```python
from build123d import *

# Parameters (mm, degrees)
BOSS_EXTRUDE1_DEPTH             = 10
SKETCH2_W                       = 1.5
SKETCH2_H                       = 4.15
TAP_DRILL_FOR_M3X0_5_TAP1_D     = 2.5
TAP_DRILL_FOR_M3X0_5_TAP1_DEPTH = 8.248924226
TAP_DRILL_FOR_M3X0_5_TAP1_TIP   = 0.751075774
CHAMFER1_SIZE                   = 2


with BuildPart() as part:
    # Sketch1 → Boss-Extrude1 (new, symmetric)
    with BuildSketch(Plane(origin=(0, 0, 0), x_dir=(1, 0, 0), z_dir=(0, 1, 0))):
        with BuildLine():
            Line((-11.8, 0), (-16.8, 0))
            Line((-16.8, 0), (-16.8, 21.8))
            Line((-16.8, 21.8), (16.8, 21.8))
            Line((16.8, 21.8), (16.8, 0))
            Line((16.8, 0), (11.8, 0))
            ThreePointArc((11.8, 0), (0, 11.8), (-11.8, 0))
        make_face()
    extrude(amount=BOSS_EXTRUDE1_DEPTH, both=True)

    # Sketch2 → Cut-Revolve1 (revolve, cut)
    with BuildSketch(Plane.XY):
        with Locations((14.3, 5)):
            Rectangle(SKETCH2_W, SKETCH2_H)
        with Locations((14.3, -5)):
            Rectangle(SKETCH2_W, SKETCH2_H)
    revolve(axis=Axis((0, 0, 0), (0, -1, 0)), mode=Mode.SUBTRACT)

    # Tap Drill for M3x0.5 Tap1
    with Locations(Plane(origin=(0, 0, -21.8), x_dir=(-1, 0, 0), z_dir=(0, 0, -1))):
        with Locations((0, 0), (11.8, -5), (11.8, 5), (-11.8, 5), (-11.8, -5)):
            Hole(TAP_DRILL_FOR_M3X0_5_TAP1_D / 2, depth=TAP_DRILL_FOR_M3X0_5_TAP1_DEPTH)
            with Locations((0, 0, -(TAP_DRILL_FOR_M3X0_5_TAP1_DEPTH + TAP_DRILL_FOR_M3X0_5_TAP1_TIP / 2))):  # 118° drill point
                Cone(0, TAP_DRILL_FOR_M3X0_5_TAP1_D / 2, TAP_DRILL_FOR_M3X0_5_TAP1_TIP, mode=Mode.SUBTRACT)

    # Chamfer1
    chamfer1_edges = [part.edges().sort_by_distance(p)[0] for p in [
        (-16.8, 0, -21.8),
        (16.8, 0, -21.8),
    ]]
    chamfer(chamfer1_edges, length=CHAMFER1_SIZE)


solid = part.part
```
Here's how the part is built. I have some questions about the finished solid (model axes, mm). A direction names the side the tool comes from. Coordinates: 2 decimals unless noted, no trailing zeros. Write each loop counter-clockwise with the first axis right and the second up, starting at its lowest first coordinate (ties: lowest second). Pieces come first, ordered by that corner, then holes. Notation, with made-up numbers: (88, -10.75) -> (112, -10.75) arc R4 ccw to (112, -4.75) -> close; hole circle Ø9 at (41.25, -16.75). An arc over 180 degrees is marked (long way). Use a Markdown table: item, result. Add a question column.
(1) If we section it at C-C, the plane x = -3: Write out the boundary of the cut face in (y, z) (3 decimals).
(2) We'd pull the mould along X, two halves only. Please class faces 4 (the cylindrical face through (-0.27, -1.22, -17.62)), 5 (the flat face through (16.8, 0, -10)), 6 (the flat face through (0, 10, -13)): +X half, -X half, draft (parallel to the pull), parting line (faces both ways), or undercut.
(3) For faces 1 (the flat face through (-16.8, 0, -10)), 2 (the flat face through (1, -2.925, -14)), 3 (the cylindrical face through (-11.223, -6.109, -17.618)), which set-ups out of +Z, -Z, +X, -X, +Y, -Y let a thin tool reach every point of the face, with its end or its side?
(4) Please list where these lines run through material, in increasing order: line 1 (X direction, y = 5, z = -17.75); line 2 (Y direction, x = -11.8, z = -19); line 3 (X direction, y = -5, z = -20).
(5) If we section it at D-D, the plane x = -11: State how many separate pieces and enclosed holes the cut face has, and give its area (3 significant figures).
(6) If we section it at B-B, the plane y = -2.25: Write out the boundary of the cut face in (x, z), and give its area (3 significant figures).
(7) I'm going to push a flat-ended pin straight in: P1, Ø2, axis at x = -11.8, y = -5, coming from the -Z side. Where does the tip first touch, or does it pass through?
(8) If we section it at A-A, the plane z = -18: Write out the boundary of the cut face in (x, y), and give its area (3 significant figures).
Outcome:
| question | item | result |
|---|---|---|
| 1 | outline | (-10, -21.8) -> (10, -21.8) -> (10, -11.412) -> (-10, -11.412) -> close; hole (-7.075, -14.748) -> (-2.925, -14.748) -> (-2.925, -13.214) -> (-7.075, -13.214) -> close; hole (2.925, -14.748) -> (7.075, -14.748) -> (7.075, -13.214) -> (2.925, -13.214) -> close |
| 2 | face 4 | undercut |
| 2 | face 5 | +X half |
| 2 | face 6 | draft |
| 3 | face 1 | +Z, -Z, -X, +Y, -Y |
| 3 | face 2 | none |
| 3 | face 3 | -Z |
| 4 | line 1 | x = -16.8 to -13.05, -10.55 to 10.55, 13.05 to 16.8 |
| 4 | line 2 | y = -10 to -6.25, -3.75 to 3.75, 6.25 to 10 |
| 4 | line 3 | x = -16.6 to -13.05, -10.55 to 10.55, 13.05 to 16.6 |
| 5 | separate pieces | 1 |
| 5 | enclosed holes | 2 |
| 5 | area | 299 mm^2 |
| 6 | outline | (-16.8, -19.8) -> (-14.8, -21.8) -> (14.8, -21.8) -> (16.8, -19.8) -> (16.8, 0) -> (11.8, 0) arc R11.8 cw to (-11.8, 0) -> (-16.8, 0) -> close |
| 6 | area | 510 mm^2 |
| 7 | P1 | stops at z = -13.4 |
| 8 | outline | (-16.8, -10) -> (16.8, -10) -> (16.8, 10) -> (-16.8, 10) -> close; hole circle Ø2.5 at (-11.8, -5); hole circle Ø2.5 at (-11.8, 5); hole circle Ø2.5 at (0, 0); hole circle Ø2.5 at (11.8, -5); hole circle Ø2.5 at (11.8, 5) |
| 8 | area | 647 mm^2 |
